Job drawing, mm, ordinate dimensions from the low corner. One solid piece. A direction names the side the tool comes from. Give positions to 0.01 mm unless a question says otherwise; leave off trailing zeros. Order: outer loops, then holes, each group sorted by start corner. A loop starts at its lowest first (then second) coordinate and runs counter-clockwise, first axis right, second up.
Item 1: Flat gauge pins, fed straight in: P1, Ø1, axis at x = 41, z = 7, coming from the -Y side; P2, Ø4, axis at x = 68, z = 5.5, coming from the -Y side; P3, Ø8, axis at x = 43.5, z = 14.5, coming from the -Y side (1 decimal). Where does each tip first touch, or does it go through?
Item 2: Band-saw the part on D-D on y = 37. Give the cut face in (x, z) (1 decimal).
Item 3: Band-saw the part on B-B on y = 80. Give the cut face in (x, z) (1 decimal).
Item 4: Which spindle directions (+Z, -Z, +X, -X, +Y, -Y) get a long thin tool onto all of the face, cutting with end or side? Do the marked faces 1, 2 and 3. Say none if no direction does.
Item 5: Wall check: L1, parallel to Z at x = 39, y = 68; L2, parallel to Z at x = 56.5, y = 24; L3, parallel to Y at x = 54.5, z = 3.25 (1 decimal). Give the ranges that are in metal, low to high.
Item 6: Band-saw the part on A-A on x = 33.5. Give the cut face in (y, z) (1 decimal), plus the area to 3 significant figures.
Item 7: Band-saw the part on C-C on z = 8.25. Give the cut face in (x, y) (1 decimal), plus the area to 3 significant figures.
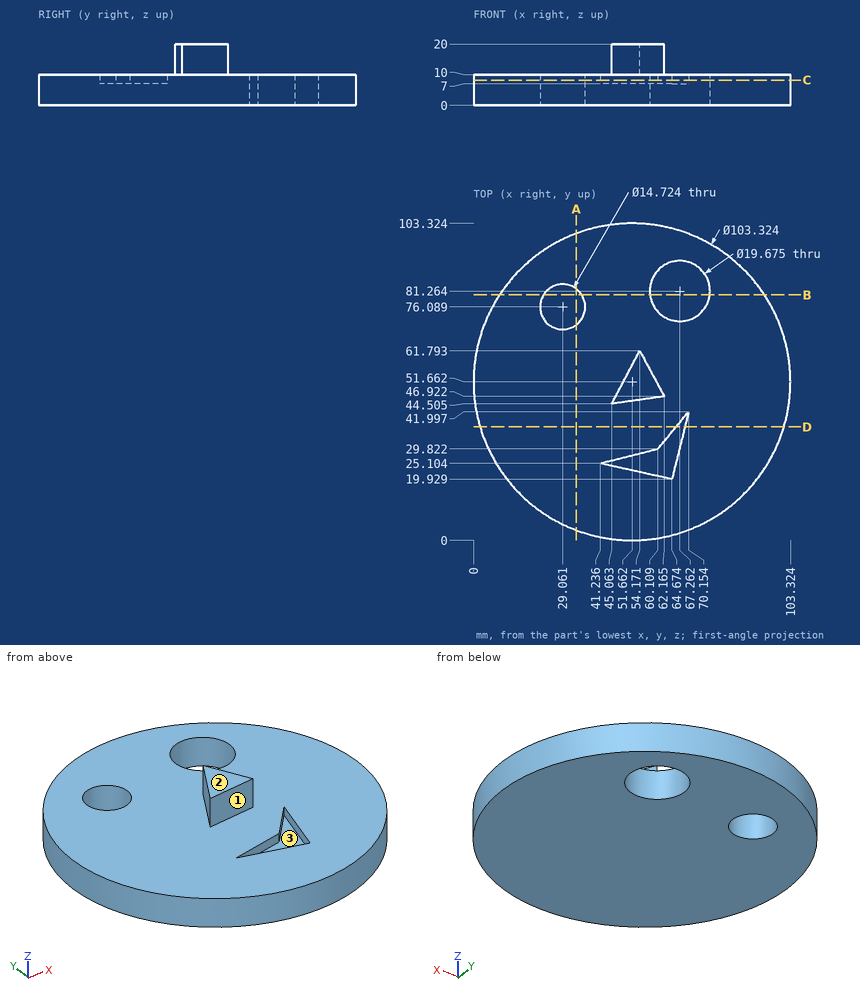
The answers:
1. P1: stops at y = 1.01
1. P2: stops at y = 2.03
1. P3: stops at y = 44.5
2. outline: (2.1, 0) - (101.2, 0) - (101.2, 10) - (68.9, 10) - (68.9, 7) - (66, 7) - (66, 10) - (2.1, 10) - close
3. outline: (8.5, 0) - (22.8, 0) - (22.8, 10) - (8.5, 10) - close; (35.3, 0) - (57.5, 0) - (57.5, 10) - (35.3, 10) - close; (77, 0) - (94.9, 0) - (94.9, 10) - (77, 10) - close
4. face 1: +Z, +X, -Y
4. face 2: +Z, +X, -X, +Y, -Y
4. face 3: +Z
5. L1: z = 0 to 10
5. L2: z = 0 to 7
5. L3: y = 0.1 to 103.2
6. outline: (3.3, 0) - (70.2, 0) - (70.2, 10) - (3.3, 10) - close; (82, 0) - (100, 0) - (100, 10) - (82, 10) - close
6. area: 850 mm2
7. outline: circle Ø103.3 at (51.7, 51.7); hole circle Ø14.7 at (29.1, 76.1); hole (41.2, 25.1) - (64.7, 19.9) - (70.2, 42) - (60.1, 29.8) - close; hole circle Ø19.7 at (67.3, 81.3)
7. area: 7,730 mm2
